Can you work these out from the model? Positions are in its coordinate system, mm. Face numbers are marked on the shaded views. A direction names the side the tool comes from. Coordinates: 2 decimals unless noted, no trailing zeros. Loops run counter-clockwise (first coordinate to the right, second up) from the corner with the lowest first, then second, coordinate; pieces in that order, holes last. Notation, with made-up numbers: (-3.75, -17) - (2.25, -17) arc R31 cw to (2.25, 10) - close; hole circle Ø11 at (74.5, 25.5). An arc over 180 degrees is marked (long way). Put each result on its own line as item: value. Start each with the question number.
from build123d import *

# Parameters (mm, degrees)
SKETCH_1_W          = 35
SKETCH_1_H          = 18.5
EXTRUDE_1_DEPTH     = 12
EXTRUDE_2_DEPTH     = 9
FILLET_1_R          = 2
CHAMFER_1_SIZE      = 1
EXTRUDE_3_DEPTH     = 1
SKETCH_4_R          = 1.825
EXTRUDE_4_DEPTH     = 6
SKETCH_5_R          = 1.2
EXTRUDE_5_DEPTH     = 15
SKETCH_6_R          = 1
CUT_EXTRUDE_1_DEPTH = 4
FILLET_2_R          = 0.3
EXTRUDE_6_DEPTH     = 0.2
FILLET_3_R          = 0.1


with BuildPart() as part:
    # 草图1 → 凸台-拉伸1 (new body)
    with BuildSketch(Plane(origin=(0, 0, 0), x_dir=(1, 0, 0), z_dir=(0, 1, 0))):
        Rectangle(SKETCH_1_W, SKETCH_1_H)
    extrude(amount=EXTRUDE_1_DEPTH)

    # 草图2 → 凸台-拉伸2 (add)
    with BuildSketch(Plane(origin=(0, 12, 0), x_dir=(1, 0, 0), z_dir=(0, 1, 0))):
        Polygon((-13, 9.25), (-17.5, 4.75), (-17.5, -4.75), (-13, -9.25), (13, -9.25), (17.5, -4.75), (17.5, 4.75), (13, 9.25), align=None)
    extrude(amount=EXTRUDE_2_DEPTH)

    # 圆角1
    fillet_1_edges = [part.edges().sort_by_distance(p)[0] for p in [
        (13, 16.5, -9.25),
        (-13, 16.5, -9.25),
        (-17.5, 16.5, -4.75),
        (-17.5, 16.5, 4.75),
        (-13, 16.5, 9.25),
        (13, 16.5, 9.25),
        (17.5, 16.5, 4.75),
        (17.5, 16.5, -4.75),
        (17.5, 6, 9.25),
        (-17.5, 6, 9.25),
        (-17.5, 6, -9.25),
        (17.5, 6, -9.25),
    ]]
    fillet(fillet_1_edges, radius=FILLET_1_R)

    # 倒角1
    chamfer_1_edges = [part.edges().sort_by_distance(p)[0] for p in [
        (0, 0, -9.25),
        (-17.5, 0, 0),
        (17.5, 0, 0),
        (0, 0, 9.25),
        (-16.914213562, 0, 8.664213562),
        (-16.914213562, 0, -8.664213562),
        (16.914213562, 0, -8.664213562),
        (16.914213562, 0, 8.664213562),
    ]]
    chamfer(chamfer_1_edges, length=CHAMFER_1_SIZE)

    # 草图3 → 凸台-拉伸3 (add)
    with BuildSketch(Plane.XY.offset(9.25)):
        with BuildLine():
            Line((-2.106, 1), (2.106, 1))
            ThreePointArc((2.106, 1), (3.395762769, 1.534237231), (3.93, 2.824))
            Line((3.93, 2.824), (3.93, 2.826))
            ThreePointArc((3.93, 2.826), (3.395762769, 4.115762769), (2.106, 4.65))
            Line((2.106, 4.65), (-2.106, 4.65))
            ThreePointArc((-2.106, 4.65), (-3.395762769, 4.115762769), (-3.93, 2.826))
            Line((-3.93, 2.826), (-3.93, 2.824))
            ThreePointArc((-3.93, 2.824), (-3.395762769, 1.534237231), (-2.106, 1))
        make_face()
    extrude(amount=EXTRUDE_3_DEPTH)

    # 草图4 → 凸台-拉伸4 (add)
    with BuildSketch(Plane.XY.offset(10.25)):
        with Locations((0, 2.825)):
            Circle(SKETCH_4_R)
    extrude(amount=EXTRUDE_4_DEPTH)

    # 草图5 → 凸台-拉伸5 (add)
    with BuildSketch(Plane.XY.offset(16.25)):
        with Locations((0, 2.825)):
            Circle(SKETCH_5_R)
    extrude(amount=EXTRUDE_5_DEPTH)

    # 草图6 → 切除-拉伸1 (cut)
    with BuildSketch(Plane.XZ):
        with Locations((-14, 5.75)):
            Circle(SKETCH_6_R)
        with Locations((14, -5.75)):
            Circle(SKETCH_6_R)
    extrude(amount=-CUT_EXTRUDE_1_DEPTH, mode=Mode.SUBTRACT)

    # 圆角2
    fillet_2_edges = [part.edges().sort_by_distance(p)[0] for p in [
        (-15, 0, 5.75),
        (13, 0, -5.75),
    ]]
    fillet(fillet_2_edges, radius=FILLET_2_R)

    # 草图7 → 凸台-拉伸6 (add)
    with BuildSketch(Plane(origin=(0, 21, 0), x_dir=(1, 0, 0), z_dir=(0, 1, 0))):
        with BuildLine():
            Line((-16.914213562, 5.335786438), (-13.585786438, 8.664213562))
            ThreePointArc((-13.585786438, 8.664213562), (-12.93693974, 9.097759065), (-12.171572875, 9.25))
            Line((-12.171572875, 9.25), (12.171572875, 9.25))
            ThreePointArc((12.171572875, 9.25), (12.93693974, 9.097759065), (13.585786438, 8.664213562))
            Line((13.585786438, 8.664213562), (16.914213562, 5.335786438))
            ThreePointArc((16.914213562, 5.335786438), (17.347759065, 4.68693974), (17.5, 3.921572875))
            Line((17.5, 3.921572875), (17.5, -3.921572875))
            ThreePointArc((17.5, -3.921572875), (17.347759065, -4.68693974), (16.914213562, -5.335786438))
            Line((16.914213562, -5.335786438), (13.585786438, -8.664213562))
            ThreePointArc((13.585786438, -8.664213562), (12.93693974, -9.097759065), (12.171572875, -9.25))
            Line((12.171572875, -9.25), (-12.171572875, -9.25))
            ThreePointArc((-12.171572875, -9.25), (-12.93693974, -9.097759065), (-13.585786438, -8.664213562))
            Line((-13.585786438, -8.664213562), (-16.914213562, -5.335786438))
            ThreePointArc((-16.914213562, -5.335786438), (-17.347759065, -4.68693974), (-17.5, -3.921572875))
            Line((-17.5, -3.921572875), (-17.5, 3.921572875))
            ThreePointArc((-17.5, 3.921572875), (-17.347759065, 4.68693974), (-16.914213562, 5.335786438))
        make_face()
        with BuildLine():
            Line((-16.560660172, 4.982233047), (-13.232233047, 8.310660172))
            ThreePointArc((-13.232233047, 8.310660172), (-12.745598024, 8.635819299), (-12.171572875, 8.75))
            Line((-12.171572875, 8.75), (-0.25, 8.75))
            Line((-0.25, 8.75), (-0.25, -8.75))
            Line((-0.25, -8.75), (-12.171572875, -8.75))
            ThreePointArc((-12.171572875, -8.75), (-12.745598024, -8.635819299), (-13.232233047, -8.310660172))
            Line((-13.232233047, -8.310660172), (-16.560660172, -4.982233047))
            ThreePointArc((-16.560660172, -4.982233047), (-16.885819299, -4.495598024), (-17, -3.921572875))
            Line((-17, -3.921572875), (-17, 3.921572875))
            ThreePointArc((-17, 3.921572875), (-16.885819299, 4.495598024), (-16.560660172, 4.982233047))
        make_face(mode=Mode.SUBTRACT)
        with BuildLine():
            Line((13.232233047, 8.310660172), (16.560660172, 4.982233047))
            ThreePointArc((16.560660172, 4.982233047), (16.885819299, 4.495598024), (17, 3.921572875))
            Line((17, 3.921572875), (17, -3.921572875))
            ThreePointArc((17, -3.921572875), (16.885819299, -4.495598024), (16.560660172, -4.982233047))
            Line((16.560660172, -4.982233047), (13.232233047, -8.310660172))
            ThreePointArc((13.232233047, -8.310660172), (12.745598024, -8.635819299), (12.171572875, -8.75))
            Line((12.171572875, -8.75), (0.25, -8.75))
            Line((0.25, -8.75), (0.25, 8.75))
            Line((0.25, 8.75), (12.171572875, 8.75))
            ThreePointArc((12.171572875, 8.75), (12.745598024, 8.635819299), (13.232233047, 8.310660172))
        make_face(mode=Mode.SUBTRACT)
    extrude(amount=EXTRUDE_6_DEPTH)

    # 圆角3
    fillet_3_edges = [part.edges().sort_by_distance(p)[0] for p in [
        (12.93693974, 21.2, -9.097759065),
        (0, 21.2, -9.25),
        (-12.93693974, 21.2, -9.097759065),
        (-15.25, 21.2, -7),
        (-17.347759065, 21.2, -4.68693974),
        (-17.5, 21.2, 0),
        (-17.347759065, 21.2, 4.68693974),
        (-15.25, 21.2, 7),
        (-12.93693974, 21.2, 9.097759065),
        (0, 21.2, 9.25),
        (12.93693974, 21.2, 9.097759065),
        (15.25, 21.2, 7),
        (17.347759065, 21.2, 4.68693974),
        (17.5, 21.2, 0),
        (17.347759065, 21.2, -4.68693974),
        (15.25, 21.2, -7),
        (-16.885819299, 21.2, -4.495598024),
        (-17, 21.2, 0),
        (-16.885819299, 21.2, 4.495598024),
        (-14.896446609, 21.2, 6.646446609),
        (-12.745598024, 21.2, 8.635819299),
        (-6.210786438, 21.2, 8.75),
        (-0.25, 21.2, 0),
        (-6.210786438, 21.2, -8.75),
        (-12.745598024, 21.2, -8.635819299),
        (-14.896446609, 21.2, -6.646446609),
        (12.745598024, 21.2, -8.635819299),
        (6.210786438, 21.2, -8.75),
        (0.25, 21.2, 0),
        (6.210786438, 21.2, 8.75),
        (12.745598024, 21.2, 8.635819299),
        (14.896446609, 21.2, 6.646446609),
        (16.885819299, 21.2, 4.495598024),
        (17, 21.2, 0),
        (16.885819299, 21.2, -4.495598024),
        (14.896446609, 21.2, -6.646446609),
    ]]
    fillet(fillet_3_edges, radius=FILLET_3_R)


solid = part.part
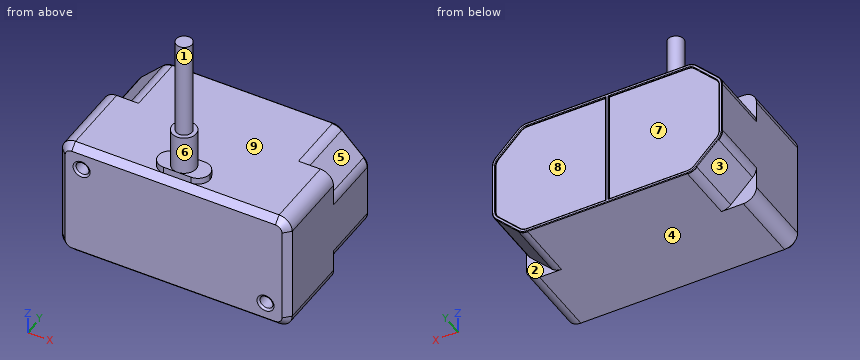
Q1. We'd pull the mould along X, two halves only. Please class the marked faces 6, 7, 8 and 9: released by +X, released by -X, zero draft, split by the parting line, or undercut.
Q2. I want a section at B-B on y = 18. List the corners of the cut face in (x, z) for me, and give its area (3 significant figures).
Q3. Please list where these lines run through material, in increasing order: line 1 along Z through (x, y) = (14, 1.45); line 2 along Z through (x, y) = (-14, 16); line 3 along Z through (x, y) = (4.5, 17.5). Write a range as [from, to].
Q4. I want a section at A-A on x = -5. List the corners of the cut face in (y, z) for me, and give its area (3 significant figures).
Q5. I want a section at C-C on y = 10.5. List the corners of the cut face in (x, z) for me, and give its area (3 significant figures).
Q6. Will these pins go through, and if not, where does the flat tip stop? pin 1 (8 mm diameter, centred on x = 4, y = 14, fed in from +Z); pin 2 (8.5 mm diameter, centred on x = 8.5, z = 1.5, fed in from +Y); pin 3 (1.2 mm diameter, centred on x = -14, z = 5.75, fed in from -Y); pin 4 (1 mm diameter, centred on y = 5.5, z = 25, fed in from +X).
Q7. On a 3-axis mill with a long thin cutter (end or side, diameter ignored), from which of +Z, -Z, +X, -X, +Y, -Y can I reach the whole of each face in a straight line? I mean the marked faces 1, 2, 3, 4 and 5. Say none if no direction works.
Q8. I want a section at D-D on z = 22. List the corners of the cut face in (x, y) for me (3 decimals).
Calculated:
1. face 6: split by the parting line
1. face 7: undercut
1. face 8: undercut
1. face 9: zero draft
2. outline: (-17.5, -3.92) arc R2 ccw to (-16.91, -5.34) - (-13.59, -8.66) arc R2 ccw to (-12.17, -9.25) - (12.17, -9.25) arc R2 ccw to (13.59, -8.66) - (16.91, -5.34) arc R2 ccw to (17.5, -3.92) - (17.5, 3.92) arc R2 ccw to (16.91, 5.34) - (13.59, 8.66) arc R2 ccw to (12.17, 9.25) - (-12.17, 9.25) arc R2 ccw to (-13.59, 8.66) - (-16.91, 5.34) arc R2 ccw to (-17.5, 3.92) - close
2. area: 606 mm2
3. line 1: [-9.25, -6.75], [-4.75, 9.25]
3. line 2: [-8.25, 8.25]
3. line 3: [-9.25, 9.25]
4. outline: (0, -8.25) - (1, -9.25) - (21.1, -9.25) arc R0.1 ccw to (21.2, -9.15) - (21.2, -8.85) arc R0.1 ccw to (21.1, -8.75) - (21, -8.75) - (21, 8.75) - (21.1, 8.75) arc R0.1 ccw to (21.2, 8.85) - (21.2, 9.15) arc R0.1 ccw to (21.1, 9.25) - (1, 9.25) - (0, 8.25) - close
4. area: 388 mm2
5. outline: (-17.5, -7.25) arc R2 ccw to (-15.5, -9.25) - (15.5, -9.25) arc R2 ccw to (17.5, -7.25) - (17.5, 7.25) arc R2 ccw to (15.5, 9.25) - (-15.5, 9.25) arc R2 ccw to (-17.5, 7.25) - close
5. area: 644 mm2
6. pin 1: z = 9.25
6. pin 2: y = 21
6. pin 3: y = 4
6. pin 4: through
7. face 1: +Z
7. face 2: -Z, +X, +Y
7. face 3: -Z, -X, +Y
7. face 4: -Z, +X, -X, +Y, -Y
7. face 5: +Z, +X, +Y
8. outline: circle Ø2.4 at (0, 2.825)
